from build123d import *
from build123d.topology import SkipClean

# Parameters (mm, degrees)
BOSS_EXTRUDE1_START = 2.2
BOSS_EXTRUDE1_DEPTH = 2.2


with BuildPart() as part:
    # Sketch2 → Revolve1 (revolve)
    with BuildSketch(Plane.XY, mode=Mode.PRIVATE) as revolve1_sk:
        Polygon((2.7, 2.2), (2.7, 1.4), (1.3, 1.4), (1.3, 0.45), (2.35, 0.45), (2.35, -2), (3.7, -2), (3.7, 2.2), align=None)
    revolve(revolve1_sk.sketch.rotate(Axis((0, 55, 0), (0, -1, 0)), 90), axis=Axis((0, 55, 0), (0, -1, 0)))

    # Sketch3 → Boss-Extrude1 (add)
    with BuildSketch(Plane(origin=(0, 0, 0), x_dir=(1, 0, 0), z_dir=(0, 1, 0)).offset(BOSS_EXTRUDE1_START)):
        with BuildLine():
            ThreePointArc((3.7, 0), (3.313087927, -1.647254803), (2.233271143, -2.95))
            Line((2.233271143, -2.95), (15.04870989, -1.994463679))
            ThreePointArc((15.04870989, -1.994463679), (13.729944749, -1.622026729), (12.960476899, -0.488108738))
            ThreePointArc((12.960476899, -0.488108738), (12.539189082, -0.389998964), (12.35208013, 0))
            Line((12.35208013, 0), (11.304160261, 0))
            ThreePointArc((11.304160261, 0), (10.804160261, -0.5), (10.304160261, 0))
            Line((10.304160261, 0), (9.256240391, 0))
            ThreePointArc((9.256240391, 0), (8.756240391, -0.5), (8.256240391, 0))
            Line((8.256240391, 0), (7.208320521, 0))
            ThreePointArc((7.208320521, 0), (6.708320521, -0.5), (6.208320521, 0))
            Line((6.208320521, 0), (5.160400652, 0))
            ThreePointArc((5.160400652, 0), (4.660400652, -0.5), (4.160400652, 0))
            Line((4.160400652, 0), (3.7, 0))
        make_face()
        with BuildLine():
            ThreePointArc((12.960476899, -0.488108738), (13.729944749, -1.622026729), (15.04870989, -1.994463679))
            ThreePointArc((15.04870989, -1.994463679), (16.36584784, -1.360621222), (16.9, 0))
            Line((16.9, 0), (15.4, 0))
            ThreePointArc((15.4, 0), (14.9, -0.5), (14.4, 0))
            Line((14.4, 0), (13.35208013, 0))
            ThreePointArc((13.35208013, 0), (13.242079095, -0.312891048), (12.960476899, -0.488108738))
        make_face()
    boss_extrude1 = extrude(amount=-BOSS_EXTRUDE1_DEPTH)

    # Mirror1: Boss-Extrude1 across plane
    with SkipClean():  # the faces are left unmerged after this step: merging them gives an invalid solid
        add(boss_extrude1.mirror(Plane(origin=(0, 17.160462404, 0), x_dir=(1, 0, 0), z_dir=(0, 0, -1))))


solid = part.part
Could you check a few things on this model? Use its own coordinates, in mm. A direction names the side the tool comes from. Round coordinates to 2 decimals unless told otherwise and drop trailing zeros. Write each loop counter-clockwise with the first axis right and the second up, starting at its lowest first coordinate (ties: lowest second). Pieces come first, ordered by that corner, then holes. Notation, with made-up numbers: (41, -26) - (62, -26) arc R21 cw to (62, 1) - close; hole circle Ø8 at (31.25, 38). An arc over 180 degrees is marked (long way). Use a Markdown table: item, result.
Q1. Please list where these lines run through material, in increasing order: L1, parallel to X at y = -0.85, z = 0; L2, parallel to Y at x = 6.25, z = 1.75; L3, parallel to X at y = -0.1, z = -0.75.
Output values:
| item | result |
|---|---|
| L1 | -3.7 to -2.35, 2.35 to 3.7 |
| L2 | 0 to 2.2 |
| L3 | -3.62 to -2.23, 2.23 to 3.62 |
Q2. I want a section at D-D (x = 10.5). List the corners of the cut face in (y, z) for me, plus the area to 3 significant figures.
Output values:
| item | result |
|---|---|
| outline | (0, -2.33) - (2.2, -2.33) - (2.2, -0.4) - (0, -0.4) - close; (0, 0.4) - (2.2, 0.4) - (2.2, 2.33) - (0, 2.33) - close |
| area | 8.52 mm2 |
Q3. I want a section at B-B (y = -0.75). List the corners of the cut face in (x, z) for me.
Output values:
| item | result |
|---|---|
| outline | circle Ø7.4 at (0, 0); hole circle Ø4.7 at (0, 0) |
Q4. I want a section at C-C (z = -1.75). List the corners of the cut face in (x, y) for me, plus the area to 3 significant figures.
Output values:
| item | result |
|---|---|
| outline | (-3.26, -2) - (-1.57, -2) - (-1.57, 0.45) - (1.57, 0.45) - (1.57, -2) - (3.26, -2) - (3.26, 0) - (15.87, 0) - (15.87, 2.2) - (2.06, 2.2) - (2.06, 1.4) - (-2.06, 1.4) - (-2.06, 2.2) - (-3.26, 2.2) - close |
| area | 44.1 mm2 |
Q5. For pin 1 (1.6 mm diameter, centred on x = -1, z = 0.5, fed in from +Y); pin 2 (1.8 mm diameter, centred on x = 11.5, z = 1.5, fed in from -Y); pin 3 (3 mm diameter, centred on x = 0, z = 0, fed in from -Y), each with a flat end and sliding along its axis, tell me the tip position at first contact or that it passes through.
Output values:
| item | result |
|---|---|
| pin 1 | y = 1.4 |
| pin 2 | y = 0 |
| pin 3 | y = 0.45 |
Q6. I want a section at A-A (x = 0). List the corners of the cut face in (y, z) for me, plus the area to 3 significant figures.
Output values:
| item | result |
|---|---|
| outline | (-2, -3.7) - (2.2, -3.7) - (2.2, -2.7) - (1.4, -2.7) - (1.4, -1.3) - (0.45, -1.3) - (0.45, -2.35) - (-2, -2.35) - close; (-2, 2.35) - (0.45, 2.35) - (0.45, 1.3) - (1.4, 1.3) - (1.4, 2.7) - (2.2, 2.7) - (2.2, 3.7) - (-2, 3.7) - close |
| area | 12.8 mm2 |
Q7. For faces 1 (the cylindrical face through (1.643, 1.794, -2.143)), 2 (the flat face through (8.55, 1.12, -2.48)), 3 (the cylindrical face through (2.294, -0.792, -0.509)), which set-ups out of +Z, -Z, +X, -X, +Y, -Y let a thin tool reach every point of the face, with its end or its side?
Output values:
| item | result |
|---|---|
| face 1 | +Y |
| face 2 | -Z, +X, +Y, -Y |
| face 3 | -Y |
